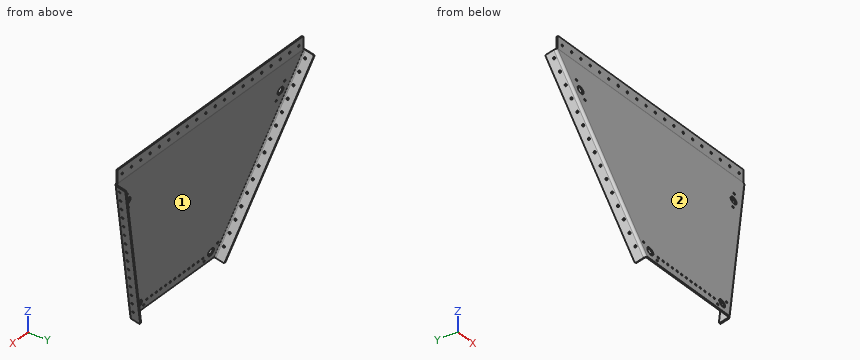
```python
from build123d import *

# Parameters (mm, degrees)
BOSS_EXTRUDE1_DEPTH             = 254
CONVERT_SOLID1_START            = -254
CONVERT_SOLID1_DEPTH            = 508
CONVERT_SOLID1_2_DEPTH          = 508
CUT_EXTRUDE1_DEPTH              = 574.396643949
EDGE_FLANGE1_DEPTH              = 393.117270957
EDGE_FLANGE1_BEND_DEPTH         = 393.117270957
SKETCH12_R                      = 7.9375
CUT_EXTRUDE2_DEPTH              = 580.286449316
F_1_4_0_25_DIAMETER_HOLE1_D     = 4.191
F_1_4_0_25_DIAMETER_HOLE1_DEPTH = 254
F_1_4_0_25_DIAMETER_HOLE1_TIP   = 1.259103427
F_1_4_0_25_DIAMETER_HOLE2_D     = 4.191
F_1_4_0_25_DIAMETER_HOLE2_DEPTH = 254
F_1_4_0_25_DIAMETER_HOLE2_TIP   = 1.259103427
F_1_4_0_25_DIAMETER_HOLE3_D     = 4.191
F_1_4_0_25_DIAMETER_HOLE3_DEPTH = 254
F_1_4_0_25_DIAMETER_HOLE3_TIP   = 1.259103427
F_1_4_0_25_DIAMETER_HOLE5_D     = 4.191
F_1_4_0_25_DIAMETER_HOLE5_DEPTH = 254
F_1_4_0_25_DIAMETER_HOLE5_TIP   = 1.259103427
SKETCH25_R                      = 2.0955
CUT_EXTRUDE3_DEPTH              = 2.54
FILLET1_R                       = 2.54


# Read off the part's stored shape, not the designer's step: Convert-Solid1
# Sheet-metal steps are written as plain solids
with BuildPart() as part:
    # Sketch3 → Boss-Extrude1 (new, symmetric)
    with BuildSketch(Plane(origin=(0, 0, 0), x_dir=(0, 0, -1), z_dir=(1, 0, 0))):
        Polygon((-477.990419123, 101.6), (-503.390419123, 101.6), (-503.390419123, 104.14), (-477.723454365, 104.14), (-118.969509086, 27.884494906), (-119.497604781, 25.4), align=None)
    extrude(amount=BOSS_EXTRUDE1_DEPTH, both=True)

    # Convert-Solid1 outline → Convert-Solid1 (cut)
    with BuildSketch(Plane.YZ.offset(CONVERT_SOLID1_START)):
        with BuildLine():
            Line((104.14, 477.723454365), (104.14, 478.257383881))
            ThreePointArc((104.14, 478.257383881), (104.112171228, 477.726379287), (104.028989812, 477.201192491))
            Line((104.028989812, 477.201192491), (104.14, 477.723454365))
        make_face()
    extrude(amount=CONVERT_SOLID1_DEPTH, mode=Mode.SUBTRACT)

    # Convert-Solid1 2 outline → Convert-Solid1 2 (add)
    with BuildSketch(Plane.YZ.offset(CONVERT_SOLID1_START)):
        with BuildLine():
            Line((101.6, 477.990419123), (101.6, 478.257383881))
            ThreePointArc((101.6, 478.257383881), (101.586085614, 477.991881584), (101.544494906, 477.729288186))
            Line((101.544494906, 477.729288186), (101.6, 477.990419123))
        make_face()
    extrude(amount=CONVERT_SOLID1_2_DEPTH)

    # Sketch8 → Cut-Extrude1 (cut, through all)
    with BuildSketch(Plane(origin=(0, 2.484494906, -0.528095695), x_dir=(1, 0, 0), z_dir=(0, 0.978147600733807, -0.20791169081775257))):
        Polygon((254, -488.402044668), (111.125, -122.167252357), (254, -122.167252357), align=None)
        Polygon((-111.125, -122.167252357), (-254, -488.402044668), (-254, -122.167252357), align=None)
    extrude(amount=-CUT_EXTRUDE1_DEPTH, mode=Mode.SUBTRACT)

    # Edge-Flange1 section (across the edge) → Edge-Flange1 (add)
    with BuildSketch(Plane(origin=(256.366307566, 103.837058096, 476.298224762), x_dir=(-0.9316171518495571, 0.07556366768945466, 0.3554991061944279), z_dir=(-0.36344116770079793, -0.19369409723586034, -0.9112590818841071))):
        with BuildLine():
            Line((-2.54, 2.54), (-2.54, 20.32))
            Line((-2.54, 20.32), (0, 20.32))
            Line((0, 20.32), (0, 2.54))
            ThreePointArc((0, 2.54), (0.743948776, 0.743948776), (2.54, 0))
            Line((2.54, 0), (2.54, -2.54))
            ThreePointArc((2.54, -2.54), (-1.052102448, -1.052102448), (-2.54, 2.54))
        make_face()
    extrude(amount=EDGE_FLANGE1_DEPTH)

    # Edge-Flange1 section 2 (across the edge) → Edge-Flange1 bend (add)
    with BuildSketch(Plane(origin=(-113.491307566, 27.69256319, 118.066541356), x_dir=(0.9316171518495615, 0.07556366768945232, 0.35549910619441694), z_dir=(-0.3634411677007866, 0.19369409723586137, 0.9112590818841114))):
        with BuildLine():
            Line((-2.54, 2.54), (-2.54, 20.32))
            Line((-2.54, 20.32), (0, 20.32))
            Line((0, 20.32), (0, 2.54))
            ThreePointArc((0, 2.54), (0.743948776, 0.743948776), (2.54, 0))
            Line((2.54, 0), (2.54, -2.54))
            ThreePointArc((2.54, -2.54), (-1.052102448, -1.052102448), (-2.54, 2.54))
        make_face()
    extrude(amount=EDGE_FLANGE1_BEND_DEPTH)

    # Sketch12 → Cut-Extrude2 (cut, symmetric)
    with BuildSketch(Plane(origin=(0, 2.484494906, -0.528095695), x_dir=(1, 0, 0), z_dir=(0, 0.978147600733807, -0.20791169081775257))):
        with Locations(Location((208.885313066, -425.17416024, 0), (0, 0, 90))):
            Circle(SKETCH12_R)
        with Locations(Location((98.108445151, -141.217252357, 0), (0, 0, 90))):
            Circle(SKETCH12_R)
    cut_extrude2 = extrude(amount=CUT_EXTRUDE2_DEPTH, both=True, mode=Mode.SUBTRACT)

    # Mirror8: Cut-Extrude2 across plane
    add(cut_extrude2.mirror(Plane(origin=(0, 0, 0), x_dir=(0, 0, 1), z_dir=(1, 0, 0))), mode=Mode.SUBTRACT)

    # 1/4 (0.25) Diameter Hole1
    with Locations(Plane(origin=(0, 104.14, 0), x_dir=(1, 0, 0), z_dir=(0, 1, 0))):
        with Locations((-241.3, -490.690419123), (-215.9, -490.690419123), (-190.5, -490.690419123), (-165.1, -490.690419123), (-139.7, -490.690419123), (-114.3, -490.690419123), (-88.9, -490.690419123), (-63.5, -490.690419123), (-38.1, -490.690419123), (-12.7, -490.690419123), (12.7, -490.690419123), (38.1, -490.690419123), (63.5, -490.690419123), (88.9, -490.690419123), (114.3, -490.690419123), (139.7, -490.690419123), (165.1, -490.690419123), (190.5, -490.690419123), (215.9, -490.690419123), (241.3, -490.690419123), (266.7, -490.690419123)):
            Hole(F_1_4_0_25_DIAMETER_HOLE1_D / 2, depth=F_1_4_0_25_DIAMETER_HOLE1_DEPTH)
            with Locations((0, 0, -(F_1_4_0_25_DIAMETER_HOLE1_DEPTH + F_1_4_0_25_DIAMETER_HOLE1_TIP / 2))):  # 118° drill point
                Cone(0, F_1_4_0_25_DIAMETER_HOLE1_D / 2, F_1_4_0_25_DIAMETER_HOLE1_TIP, mode=Mode.SUBTRACT)

    # 1/4 (0.25) Diameter Hole2
    with Locations(Plane(origin=(59.814802644, -4.851591516, -22.824943524), x_dir=(-0.35412064344222605, 0.031373259319903056, -0.9346733592478765), z_dir=(0.9316171518495572, -0.07556366768945416, -0.3554991061944278))):
        with Locations((-518.621219682, 130.197638553), (-493.872607959, 124.482201754), (-469.123996237, 118.766764955), (-444.375384514, 113.051328156), (-419.626772792, 107.335891357), (-394.878161069, 101.620454558), (-370.129549346, 95.905017759), (-345.380937624, 90.18958096), (-320.632325901, 84.474144161), (-295.883714179, 78.758707362), (-271.135102456, 73.043270563), (-246.386490734, 67.327833764), (-221.637879011, 61.612396964), (-196.889267288, 55.896960165), (-172.140655566, 50.181523366)):
            Hole(F_1_4_0_25_DIAMETER_HOLE2_D / 2, depth=F_1_4_0_25_DIAMETER_HOLE2_DEPTH)
            with Locations((0, 0, -(F_1_4_0_25_DIAMETER_HOLE2_DEPTH + F_1_4_0_25_DIAMETER_HOLE2_TIP / 2))):  # 118° drill point
                Cone(0, F_1_4_0_25_DIAMETER_HOLE2_D / 2, F_1_4_0_25_DIAMETER_HOLE2_TIP, mode=Mode.SUBTRACT)

    # 1/4 (0.25) Diameter Hole3
    with Locations(Plane(origin=(-59.814802644, -4.851591516, -22.824943524), x_dir=(-0.3541206434422149, -0.03137325931990071, 0.9346733592478808), z_dir=(-0.9316171518495615, -0.07556366768945355, -0.3554991061944165))):
        with Locations((518.621219682, 130.197638553), (493.872607959, 124.482201754), (469.123996237, 118.766764955), (444.375384514, 113.051328156), (419.626772792, 107.335891357), (394.878161069, 101.620454558), (370.129549346, 95.905017759), (345.380937624, 90.18958096), (320.632325901, 84.474144161), (295.883714179, 78.758707362), (271.135102456, 73.043270563), (246.386490734, 67.327833764), (221.637879011, 61.612396964), (196.889267288, 55.896960165), (172.140655566, 50.181523366)):
            Hole(F_1_4_0_25_DIAMETER_HOLE3_D / 2, depth=F_1_4_0_25_DIAMETER_HOLE3_DEPTH)
            with Locations((0, 0, -(F_1_4_0_25_DIAMETER_HOLE3_DEPTH + F_1_4_0_25_DIAMETER_HOLE3_TIP / 2))):  # 118° drill point
                Cone(0, F_1_4_0_25_DIAMETER_HOLE3_D / 2, F_1_4_0_25_DIAMETER_HOLE3_TIP, mode=Mode.SUBTRACT)

    # 1/4 (0.25) Diameter Hole5
    with Locations(Plane(origin=(0, 2.484494906, -0.528095695), x_dir=(1, 0, 0), z_dir=(0, 0.9781476007338071, -0.2079116908177526))):
        with Locations((76.2, -139.814560704), (63.5, -139.814560704), (50.8, -139.814560704), (38.1, -139.814560704), (25.4, -139.814560704), (12.7, -139.814560704), (0, -139.814560704), (-12.7, -139.814560704), (-25.4, -139.814560704), (-38.1, -139.814560704), (-50.8, -139.814560704), (-63.5, -139.814560704), (-76.2, -139.814560704)):
            Hole(F_1_4_0_25_DIAMETER_HOLE5_D / 2, depth=F_1_4_0_25_DIAMETER_HOLE5_DEPTH)
            with Locations((0, 0, -(F_1_4_0_25_DIAMETER_HOLE5_DEPTH + F_1_4_0_25_DIAMETER_HOLE5_TIP / 2))):  # 118° drill point
                Cone(0, F_1_4_0_25_DIAMETER_HOLE5_D / 2, F_1_4_0_25_DIAMETER_HOLE5_TIP, mode=Mode.SUBTRACT)

    # Sketch25 → Cut-Extrude3 (cut)
    with BuildSketch(Plane(origin=(0, 2.484494906, -0.528095695), x_dir=(1, 0, 0), z_dir=(0, 0.9781476007338071, -0.2079116908177526))):
        with Locations(Location((-215.248775979, -443.13558852, 0), (0, 0, 270))):
            Circle(SKETCH25_R)
        with Locations(Location((-202.139295591, -407.361973607, 0), (0, 0, 270))):
            Circle(SKETCH25_R)
        with Locations(Location((-113.372717488, -152.428680891, 0), (0, 0, 270))):
            Circle(SKETCH25_R)
        with Locations(Location((-82.461618252, -130.155065468, 0), (0, 0, 270))):
            Circle(SKETCH25_R)
    cut_extrude3 = extrude(amount=-CUT_EXTRUDE3_DEPTH, mode=Mode.SUBTRACT)

    # Mirror9: Cut-Extrude3 across plane
    add(cut_extrude3.mirror(Plane(origin=(0, 0, 0), x_dir=(0, 0, 1), z_dir=(1, 0, 0))), mode=Mode.SUBTRACT)

    # Fillet1
    fillet1_edges = [part.edges().sort_by_distance(p)[0] for p in [
        (254, 102.87, 503.390419123),
        (-254, 102.87, 503.390419123),
        (257.549461349, 123.617051485, 471.621975339),
        (114.674461349, 47.472556579, 113.390291934),
        (-114.674461349, 47.472556579, 113.390291934),
        (-257.549461349, 123.617051485, 471.621975339),
    ]]
    fillet(fillet1_edges, radius=FILLET1_R)


solid = part.part
```
Verification items for the finished model (mm, model axes). Face numbers are marked on the shaded views. Give positions to 0.01 mm unless a question says otherwise; leave off trailing zeros. Return JSON: item names as keys, results as strings. Group by question number.
1) Go/stop test with flat-tipped pins: pin 1 Ø3 at (x, z) = (61, 173.5) entering from +Y; pin 2 Ø7.5 at (x, z) = (97, 488.5) entering from -Y; pin 3 Ø6.5 at (x, z) = (88.9, 490.69) entering from +Y. Record where each tip stops, or that it passes through.
2) Mould release check, pull along Z, two halves, no side actions. Record for the marked faces 1 and 2: pulls with the +Z half, pulls with the -Z half, needs draft (parallel to the pull), parting line crosses it, or undercut.
3) Scan lines: line 1 (X direction, y = 61, z = 257); line 2 (Y direction, x = 64, z = 391); line 3 (Y direction, x = -152, z = 461). Record each from-to range of solid material in increasing order.
Answer block:
{
 "1": {"pin 1": "stops at y = 39.79", "pin 2": "stops at y = 101.6", "pin 3": "stops at y = 104.14"},
 "2": {"face 1": "undercut", "face 2": "pulls with the +Z half"},
 "3": {"line 1": "x = -171.94 to -169.21, 169.21 to 171.94", "line 2": "y = 83.11 to 85.71", "line 3": "y = 97.99 to 100.59"}
}
